Source: CAD feature listing. Evaluate the final solid. Frame: model axes, mm. A direction names the side the tool comes from. Round coordinates to 2 decimals unless told otherwise and drop trailing zeros. Loops run counter-clockwise (first coordinate to the right, second up) from the corner with the lowest first, then second, coordinate; pieces in that order, holes last.
(1) Material intervals for probe 1 along Y at (x, z) = (0, 18.25); probe 2 along Z at (x, y) = (26, -4); probe 3 along Z at (x, y) = (-22.5, -8.5), sorted ascending.
(2) Section C-C, the plane y = -3.5. Return the cut outline in (x, z).
(3) Section A-A, the plane x = -20. Return the cut outline in (y, z), plus the area to 3 significant figures.
(4) Section D-D, the plane x = 4. Return the cut outline in (y, z), plus the area to 3 significant figures.
(5) Mould query, pull axis Y, two halves, no side actions, for faces 1 (the cylindrical face through (14, -2, 12)), 2 (the cylindrical face through (-7.167, 4.57, 11.339)), 3 (the cylindrical face through (-17.507, 17.846, 8.07)), 4 (the cylindrical face through (-17.846, -17.507, 8.07)). Classes: pulls with the +Y half, pulls with the -Y half, needs draft (parallel to the pull), parting line crosses it, or undercut.
(6) First-contact query: pin 1 Ø2 at (y, z) = (16, 10) entering from -X; pin 2 Ø10.5 at (y, z) = (22.5, 3.5) entering from -X; pin 3 Ø1 at (x, y) = (9.5, 22.5) entering from -Z; pin 4 Ø6 at (x, z) = (24.5, 13) entering from +Y. Flat tips, straight axial feed; report the tip coordinate or a pass-through.
(7) Set-up query: faces 5 (the cylindrical face through (-10.51, 10.7, 18.07)), 6 (the cylindrical face through (2, -14, 12)), 7 (the flat face through (18, 18, 3)), 8 (the flat face through (18, -18, 3)), 9 (the cylindrical face through (-14, 2, 12)). Return all of +Z, -Z, +X, -X, +Y, -Y with unobstructed straight access to the full face (end or side cutting, diameter ignored); none if empty.
```python
from build123d import *

# Parameters (mm, degrees)
F3_DEPTH = 23.001
F4_R     = 2.5
F4_R_2   = 2.49999


# Not quite as in the source:
# - a fillet or chamfer is up to 0.001 mm smaller than in the source, because OpenCascade refuses the exact size


with BuildPart() as f1:
    # F0 (on Right) → F1 (revolve)
    with BuildSketch(Plane.YZ):
        Polygon((8.5, 23), (8.5, 0), (32, 0), (32, 3), (25, 3), (25, 13), (15, 13), (15, 23), align=None)
    revolve(axis=Axis((0, 0, 31.7647196352), (0, 0, 1)))

    # F2 (on face) → F3 (cut, through all)
    with BuildSketch(Plane(origin=(0, 0, 0), x_dir=(1, 0, 0), z_dir=(0, 0, -1))):
        with BuildLine():
            Line((-2.5, 13), (2.5, 13))
            Line((2.5, 13), (2.5, 31.9021942819))
            ThreePointArc((2.5, 31.9021942819), (0, 32), (-2.5, 31.9021942819))
            Line((-2.5, 31.9021942819), (-2.5, 13))
        make_face()
        with BuildLine():
            ThreePointArc((32, 0), (31.9755392216, 1.2509562301), (31.9021942819, 2.5))
            Line((31.9021942819, 2.5), (13, 2.5))
            Line((13, 2.5), (13, -2.5))
            Line((13, -2.5), (31.9021942819, -2.5))
            ThreePointArc((31.9021942819, -2.5), (31.9755392216, -1.2509562301), (32, 0))
        make_face()
        with BuildLine():
            Line((-2.5, -13), (-2.5, -31.9021942819))
            ThreePointArc((-2.5, -31.9021942819), (0, -32), (2.5, -31.9021942819))
            Line((2.5, -31.9021942819), (2.5, -13))
            Line((2.5, -13), (-2.5, -13))
        make_face()
        with BuildLine():
            Line((-13, 2.5), (-31.9021942819, 2.5))
            ThreePointArc((-31.9021942819, 2.5), (-32, 0), (-31.9021942819, -2.5))
            Line((-31.9021942819, -2.5), (-13, -2.5))
            Line((-13, -2.5), (-13, 2.5))
        make_face()
    extrude(amount=-F3_DEPTH, mode=Mode.SUBTRACT)

    # F4 (call 1 of 8: OpenCascade refuses the feature's edges together)
    f4_edges = [f1.edges().sort_by_distance(p)[0] for p in [
        (-2.5, -13, 11.5),
    ]]
    fillet(f4_edges, radius=F4_R)

    # F4#2 (call 2 of 8) (radius 2.5 in the source; OpenCascade refuses exactly that, so slightly less here)
    f4_2_edges = [f1.edges().sort_by_distance(p)[0] for p in [
        (2.5, -13, 11.5),
    ]]
    fillet(f4_2_edges, radius=F4_R_2)

    # F4#3 (call 3 of 8)
    f4_3_edges = [f1.edges().sort_by_distance(p)[0] for p in [
        (13, -2.5, 11.5),
    ]]
    fillet(f4_3_edges, radius=F4_R)

    # F4#4 (call 4 of 8) (radius 2.5 in the source; OpenCascade refuses exactly that, so slightly less here)
    f4_4_edges = [f1.edges().sort_by_distance(p)[0] for p in [
        (13, 2.5, 11.5),
    ]]
    fillet(f4_4_edges, radius=F4_R_2)

    # F4#5 (call 5 of 8)
    f4_5_edges = [f1.edges().sort_by_distance(p)[0] for p in [
        (-2.5, 13, 11.5),
    ]]
    fillet(f4_5_edges, radius=F4_R)

    # F4#6 (call 6 of 8) (radius 2.5 in the source; OpenCascade refuses exactly that, so slightly less here)
    f4_6_edges = [f1.edges().sort_by_distance(p)[0] for p in [
        (2.5, 13, 11.5),
    ]]
    fillet(f4_6_edges, radius=F4_R_2)

    # F4#7 (call 7 of 8)
    f4_7_edges = [f1.edges().sort_by_distance(p)[0] for p in [
        (-13, 2.5, 11.5),
    ]]
    fillet(f4_7_edges, radius=F4_R)

    # F4#8 (call 8 of 8) (radius 2.5 in the source; OpenCascade refuses exactly that, so slightly less here)
    f4_8_edges = [f1.edges().sort_by_distance(p)[0] for p in [
        (-13, -2.5, 11.5),
    ]]
    fillet(f4_8_edges, radius=F4_R_2)


solid = f1.part
```
Output values:
1. probe 1: y = -13 to -8.5, 8.5 to 13
1. probe 2: z = 0 to 3
1. probe 3: z = 0 to 13
2. outline: (-31.81, 0) - (-7.75, 0) - (-7.75, 23) - (-14.59, 23) - (-14.59, 13) - (-24.75, 13) - (-24.75, 3) - (-31.81, 3) - close; (7.75, 0) - (31.81, 0) - (31.81, 3) - (24.75, 3) - (24.75, 13) - (14.59, 13) - (14.59, 23) - (7.75, 23) - close
3. outline: (-24.98, 0) - (-2.5, 0) - (-2.5, 13) - (-15, 13) - (-15, 3) - (-24.98, 3) - close; (2.5, 0) - (24.98, 0) - (24.98, 3) - (15, 3) - (15, 13) - (2.5, 13) - close
3. area: 385 mm2
4. outline: (-31.75, 0) - (-7.5, 0) - (-7.5, 23) - (-14.46, 23) - (-14.46, 13) - (-24.68, 13) - (-24.68, 3) - (-31.75, 3) - close; (7.5, 0) - (31.75, 0) - (31.75, 3) - (24.68, 3) - (24.68, 13) - (14.46, 13) - (14.46, 23) - (7.5, 23) - close
4. area: 628 mm2
5. face 1: undercut
5. face 2: undercut
5. face 3: pulls with the +Y half
5. face 4: pulls with the -Y half
6. pin 1: stops at x = -20
6. pin 2: stops at x = -26.94
6. pin 3: stops at z = 0
6. pin 4: stops at y = 12.76
7. face 5: +Z, -X, +Y
7. face 6: +Z, -Z, -Y
7. face 7: +Z, +X, +Y
7. face 8: +Z, +X, -Y
7. face 9: +Z, -Z, -X
